Here's how the part is built. I have some questions about the finished solid (model axes, mm). A direction names the side the tool comes from. Coordinates: 2 decimals unless noted, no trailing zeros. Write each loop counter-clockwise with the first axis right and the second up, starting at its lowest first coordinate (ties: lowest second). Pieces come first, ordered by that corner, then holes. Notation, with made-up numbers: M 42.5,-8 L 95.5,-8 A11 ccw 95.5,5 Z; hole C 63,62.25 d3. An arc over 180 degrees is marked long. Use one line per item in the form item = value. Start each with the question number.
1. I want a section at C-C, the plane y = -43.5. List the corners of the cut face in (x, z) for me (3 decimals).
2. I want a section at D-D, the plane z = -0.8. Count the separate pieces of the cut face and the enclosed holes in it, plus the area to 3 significant figures.
3. I want a section at B-B, the plane x = 0. List the corners of the cut face in (y, z) for me (3 decimals), plus the area to 3 significant figures.
4. Thinking about a two-plate mould opening in Y: for faces 1 (the face through (18.14, -47.6, -0.02)), 2 (the face through (15.455, -43.958, -0.021)), 3 (the face through (-6, -18, 1.5)), which applies, released by +Y, released by -Y, zero draft, split by the parting line, or undercut?
5. Please list where these lines run through material, in increasing order: line 1 along X through (y, z) = (-43.5, 0.3) (3 decimals); line 2 along X through (y, z) = (-16.5, -1.3); line 3 along Y through (x, z) = (-14, -0.7) (3 decimals). Write a range as [from, to].
6. On a 3-axis mill with a long thin cutter (end or side, diameter ignored), from which of +Z, -Z, +X, -X, +Y, -Y can I reach the whole of each face in a straight line? I mean faces 4 (the face through (-19, -33, 0)), 5 (the face through (19.43, 0.61, 0.02)). Say none if no direction works.
7. I want a section at A-A, the plane y = 0. List the corners of the cut face in (x, z) for me (3 decimals), plus the area to 3 significant figures.
from build123d import *

# Parameters (mm, degrees)
SKETCH_1_R          = 27.5
SKETCH_1_R_2        = 13.05
EXTRUDE_1_DEPTH     = 1.5
SKETCH_2_R          = 2.025
CUT_EXTRUDE_1_DEPTH = 17
EXTRUDE_2_DEPTH     = 3
SKETCH_5_R          = 1.525
CUT_EXTRUDE_2_DEPTH = 3
FILLET_1_R          = 3
SKETCH_7_R          = 1.525
CUT_EXTRUDE_4_DEPTH = 5


with BuildPart() as part:
    # 草图1 → 凸台-拉伸1 (new, symmetric)
    with BuildSketch(Plane.XY):
        Circle(SKETCH_1_R)
        Circle(SKETCH_1_R_2, mode=Mode.SUBTRACT)
    extrude(amount=EXTRUDE_1_DEPTH, both=True)

    # 草图2 → 切除-拉伸1 (cut, symmetric)
    with BuildSketch(Plane.XY.offset(1.5)):
        with Locations((0, 17.5)):
            Circle(SKETCH_2_R)
        with Locations((12.374368671, 12.374368671)):
            Circle(SKETCH_2_R)
        with Locations((17.5, 0)):
            Circle(SKETCH_2_R)
        with Locations((12.374368671, -12.374368671)):
            Circle(SKETCH_2_R)
        with Locations((0, -17.5)):
            Circle(SKETCH_2_R)
        with Locations((-12.374368671, -12.374368671)):
            Circle(SKETCH_2_R)
        with Locations((-17.5, 0)):
            Circle(SKETCH_2_R)
        with Locations((-12.374368671, 12.374368671)):
            Circle(SKETCH_2_R)
    extrude(amount=CUT_EXTRUDE_1_DEPTH, both=True, mode=Mode.SUBTRACT)

    # 草图4 → 凸台-拉伸2 (add)
    with BuildSketch(Plane.XY.offset(1.5)):
        with BuildLine():
            Line((-19, -19.880895352), (-19, -48.5))
            Line((-19, -48.5), (19, -48.5))
            Line((19, -48.5), (19, -19.880895352))
            ThreePointArc((19, -19.880895352), (0, -27.5), (-19, -19.880895352))
        make_face()
    extrude(amount=-EXTRUDE_2_DEPTH)

    # 草图5 → 切除-拉伸2 (cut)
    with BuildSketch(Plane(origin=(0, 0, -1.5), x_dir=(-1, 0, 0), z_dir=(0, 0, -1))):
        with Locations((17.324116139, 17.324116139)):
            Circle(SKETCH_5_R)
        with Locations((17.324116139, -17.324116139)):
            Circle(SKETCH_5_R)
        with Locations((-17.324116139, -17.324116139)):
            Circle(SKETCH_5_R)
        with Locations((-17.324116139, 17.324116139)):
            Circle(SKETCH_5_R)
    extrude(amount=-CUT_EXTRUDE_2_DEPTH, mode=Mode.SUBTRACT)

    # 圆角1
    fillet_1_edges = [part.edges().sort_by_distance(p)[0] for p in [
        (-19, -19.880895352, 0),
        (19, -19.880895352, 0),
        (19, -48.5, 0),
        (-19, -48.5, 0),
    ]]
    fillet(fillet_1_edges, radius=FILLET_1_R)

    # 草图7 → 切除-拉伸4 (cut, symmetric)
    with BuildSketch(Plane(origin=(0, 0, -1.5), x_dir=(-1, 0, 0), z_dir=(0, 0, -1))):
        with Locations(Location((-14, -43.5, 0), (0, 0, 180))):
            Circle(SKETCH_7_R)
        with Locations(Location((-14, -28.5, 0), (0, 0, 180))):
            Circle(SKETCH_7_R)
        with Locations(Location((14, -43.5, 0), (0, 0, 180))):
            Circle(SKETCH_7_R)
        with Locations(Location((14, -28.5, 0), (0, 0, 180))):
            Circle(SKETCH_7_R)
    extrude(amount=CUT_EXTRUDE_4_DEPTH, both=True, mode=Mode.SUBTRACT)


solid = part.part
Answer list:
q1.outline = M -19,-1.5 L -15.525,-1.5 L -15.525,1.5 L -19,1.5 Z; M -12.475,-1.5 L 12.475,-1.5 L 12.475,1.5 L -12.475,1.5 Z; M 15.525,-1.5 L 19,-1.5 L 19,1.5 L 15.525,1.5 Z
q2.separate_pieces = 1
q2.enclosed_holes = 17
q2.area = 2,560 mm²
q3.outline = M -48.5,-1.5 L -19.525,-1.5 L -19.525,1.5 L -48.5,1.5 Z; M -15.475,-1.5 L -13.05,-1.5 L -13.05,1.5 L -15.475,1.5 Z; M 13.05,-1.5 L 15.475,-1.5 L 15.475,1.5 L 13.05,1.5 Z; M 19.525,-1.5 L 27.5,-1.5 L 27.5,1.5 L 19.525,1.5 Z
q3.area = 125 mm²
q4.face_1 = released by -Y
q4.face_2 = undercut
q4.face_3 = zero draft
q5.line_1 = [-19, -15.525], [-12.475, 12.475], [15.525, 19]
q5.line_2 = [-22, -18.61], [-16.04, -1.76], [1.76, 16.04], [18.61, 22]
q5.line_3 = [-48.5, -45.025], [-41.975, -30.025], [-26.975, -13.582], [-11.167, 11.167], [13.582, 23.67]
q6.face_4 = +Z, -Z, -X, -Y
q6.face_5 = +Z, -Z
q7.outline = M -27.5,-1.5 L -19.525,-1.5 L -19.525,1.5 L -27.5,1.5 Z; M -15.475,-1.5 L -13.05,-1.5 L -13.05,1.5 L -15.475,1.5 Z; M 13.05,-1.5 L 15.475,-1.5 L 15.475,1.5 L 13.05,1.5 Z; M 19.525,-1.5 L 27.5,-1.5 L 27.5,1.5 L 19.525,1.5 Z
q7.area = 62.4 mm²
